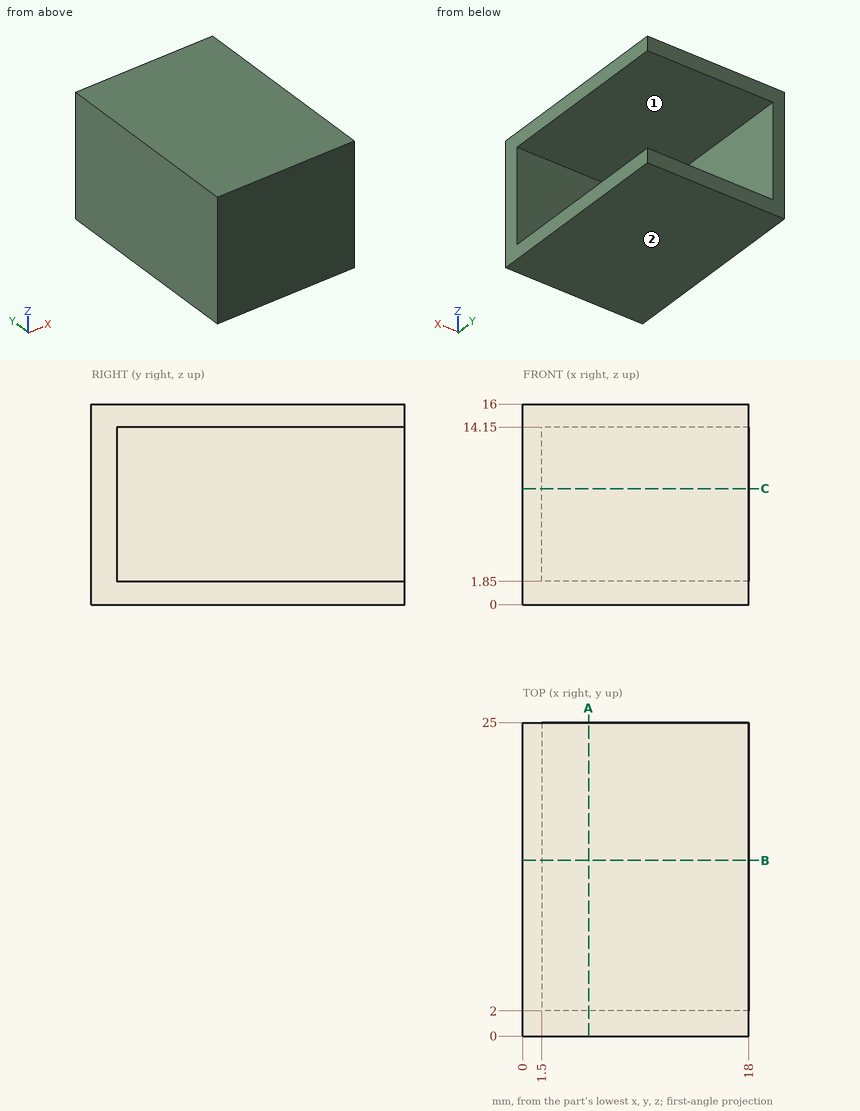
The drawing under review shows one solid part. Ordinate dimensions are in mm from its lowest x, y, z. A direction names the side the tool comes from. Give positions to 0.01 mm unless a question says otherwise; leave off trailing zeros. Order: outer loops, then holes, each group sorted by start corner. A loop starts at its lowest first (then second) coordinate and runs counter-clockwise, first axis right, second up. Notation, with made-up numbers: M 6,73.5 L 17,73.5 A20 ccw 17,89.5 Z; hole C 11,-8 d7. An arc over 180 degrees is marked long. One line per question, with ' | ' between items. Start each with the question number.
Q1. For pin 1 Ø1.5 at (y, z) = (8.5, 11.5) entering from +X; pin 2 Ø6 at (x, z) = (8, 10.5) entering from +Y, all flat-tipped, find the tip position at first contact; note any pin that passes through.
Q2. We need section B-B (y = 14). Write out the cut boundary in (x, z), plus the area to 4 significant figures.
Q3. Machinability: for the marked faces 1 and 2, which of the approach directions +Z, -Z, +X, -X, +Y, -Y give a long, thin tool a straight path to every point of the face, cutting with its end or side? Answer none if there is none.
Q4. For L1, parallel to Z at x = 15, y = 10.75; L2, parallel to Y at x = 4.25, z = 11.5; L3, parallel to X at y = 23.5, z = 11, list the stretches that pass through material, from the lowest coordinate up. Write a range as [from, to].
Q5. We need section C-C (z = 9.25). Write out the cut boundary in (x, y).
Q6. We need section A-A (x = 5.25). Write out the cut boundary in (y, z), plus the area to 3 significant figures.
Returned:
1) pin 1: x = 1.5 | pin 2: y = 2
2) outline: M 0,0 L 18,0 L 18,1.85 L 1.5,1.85 L 1.5,14.15 L 18,14.15 L 18,16 L 0,16 Z | area: 85.05 mm2
3) face 1: +X, +Y | face 2: -Z, +X, -X, +Y, -Y
4) L1: [0, 1.85], [14.15, 16] | L2: [0, 2] | L3: [0, 1.5]
5) outline: M 0,0 L 18,0 L 18,2 L 1.5,2 L 1.5,25 L 0,25 Z
6) outline: M 0,0 L 25,0 L 25,1.85 L 2,1.85 L 2,14.15 L 25,14.15 L 25,16 L 0,16 Z | area: 117 mm2
